Could you check a few things on this drawing? It's one solid part, dimensions in mm from its lowest x, y, z. A direction names the side the tool comes from. Give positions to 0.01 mm unless a question says otherwise; leave off trailing zeros. Loops run counter-clockwise (first coordinate to the right, second up) from the corner with the lowest first, then second, coordinate; pieces in that order, holes last. Notation, with made-up numbers: (-9.75, -25) - (4.25, -25) arc R14 cw to (4.25, -16) - close; hole circle Ø10 at (-16, 80). An arc over 180 degrees is marked (long way). Use CSV: the item, a comma, the result in double quotes.
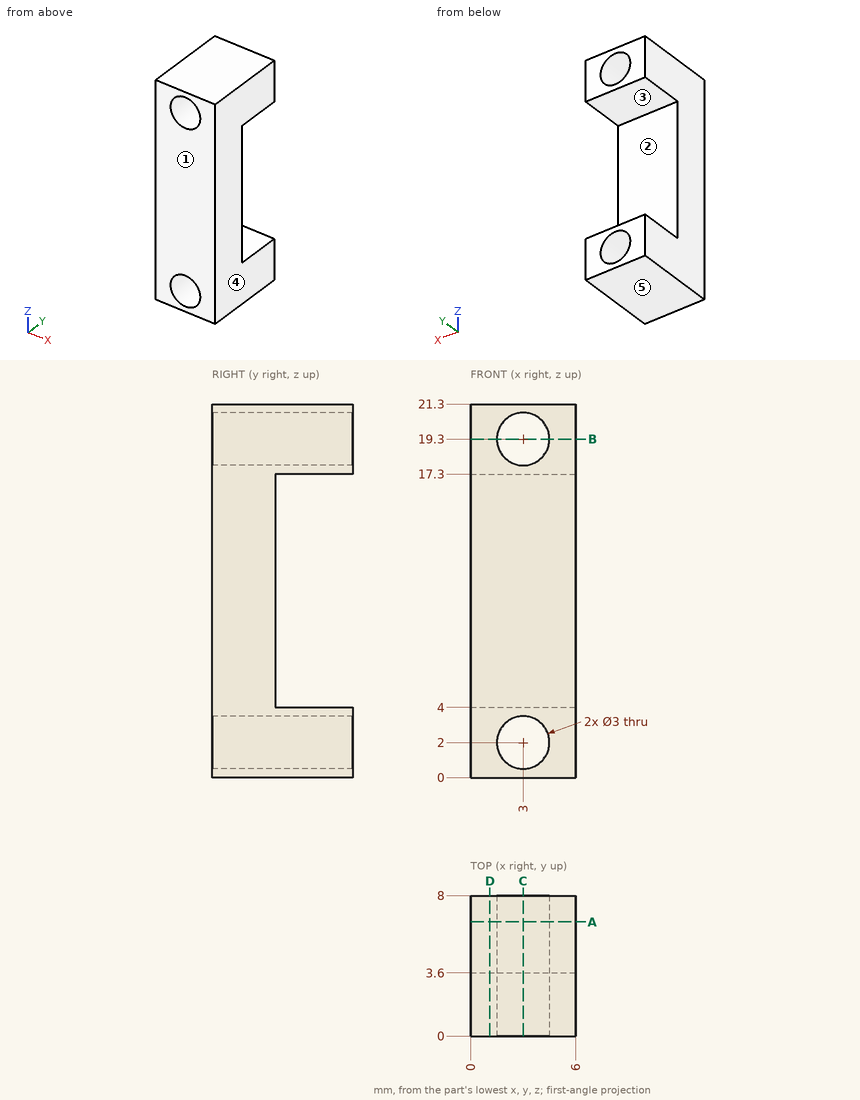
1) Suppose I cut it at D-D (x = 1.1). Please give me the cut outline in (y, z), plus the area to 3 significant figures.
Answer below:
outline,"(0, 0) - (8, 0) - (8, 4) - (3.6, 4) - (3.6, 17.3) - (8, 17.3) - (8, 21.3) - (0, 21.3) - close"
area,"112 mm2"
2) Suppose I cut it at B-B (z = 19.3). Please give me the cut outline in (x, y), plus the area to 3 significant figures.
Answer below:
outline,"(0, 0) - (1.5, 0) - (1.5, 8) - (0, 8) - close; (4.5, 0) - (6, 0) - (6, 8) - (4.5, 8) - close"
area,"24.0 mm2"
3) Which directions (+Z, -Z, +X, -X, +Y, -Y) give clear straight access to the entire face, cutting with the end or side of a thin tool? Please do the marked faces 1 and 2.
Answer below:
face 1,"+Z, -Z, +X, -X, -Y"
face 2,"+X, -X, +Y"
4) Suppose I cut it at A-A (y = 6.5). Please give me the cut outline in (x, z).
Answer below:
outline,"(0, 0) - (6, 0) - (6, 4) - (0, 4) - close; (0, 17.3) - (6, 17.3) - (6, 21.3) - (0, 21.3) - close; hole circle Ø3 at (3, 2); hole circle Ø3 at (3, 19.3)"
5) Suppose I cut it at C-C (x = 3). Please give me the cut outline in (y, z), plus the area to 3 significant figures.
Answer below:
outline,"(0, 0) - (8, 0) - (8, 0.5) - (0, 0.5) - close; (0, 3.5) - (8, 3.5) - (8, 4) - (3.6, 4) - (3.6, 17.3) - (8, 17.3) - (8, 17.8) - (0, 17.8) - close; (0, 20.8) - (8, 20.8) - (8, 21.3) - (0, 21.3) - close"
area,"63.9 mm2"
6) I need wall thicknesses on line 1 along Z through (x, y) = (3.8, 6.5); line 2 along Z through (x, y) = (0.75, 4.75); line 3 along Y through (x, z) = (2.55, 6.5). Which ranges of each line are inside material? Lowest first, please.
Answer below:
line 1,"z = 0 to 0.73, 3.27 to 4, 17.3 to 18.03, 20.57 to 21.3"
line 2,"z = 0 to 4, 17.3 to 21.3"
line 3,"y = 0 to 3.6"
7) I'm going to push flat-ended pins straight in: P1, Ø3.5, axis at x = 3.5, y = 7, coming from the -Z side; P2, Ø3, axis at x = 2.5, z = 13, coming from the +Y side. Where does each tip first touch, or does it pass through?
Answer below:
P1,"stops at z = 0"
P2,"stops at y = 3.6"
8) We'd pull the mould along Z, two halves only. Please class the marked faces 3, 4 and 5: +Z half, -Z half, draft (parallel to the pull), parting line (faces both ways), or undercut.
Answer below:
face 3,"undercut"
face 4,"draft"
face 5,"-Z half"
